Design review of the part built by this model. Coordinates are the model's own, in mm. Give positions to 0.01 mm unless a question says otherwise; leave off trailing zeros. Order: outer loops, then holes, each group sorted by start corner. A loop starts at its lowest first (then second) coordinate and runs counter-clockwise, first axis right, second up.
```python
from build123d import *

# Parameters (mm, degrees)
SKICA1_R                     = 76.5
P_IDAT_VYSUNUT_M1_DEPTH      = 20
P_IDAT_VYSUNUT_M1_DEPTH_BACK = 6.6
ODEBRAT_VYSUNUT_M1_DEPTH     = 5
ZAOBLIT1_R                   = 2
ZAOBLIT2_R                   = 5


with BuildPart() as part:
    # Skica1 → Přidat vysunutím1 (new body, two sides)
    with BuildSketch(Plane.XY) as p_idat_vysunut_m1_sk:
        Circle(SKICA1_R)
    extrude(amount=P_IDAT_VYSUNUT_M1_DEPTH)
    extrude(p_idat_vysunut_m1_sk.sketch, amount=-P_IDAT_VYSUNUT_M1_DEPTH_BACK)

    # Skica2 → Odebrat vysunutím1 (cut)
    with BuildSketch(Plane(origin=(0, 0, -6.6), x_dir=(-1, 0, 0), z_dir=(0, 0, -1))):
        Polygon((25, -10), (48.8, -10), (48.8, 10), (25, 10), (25, 25), (10, 25), (10, 48.8), (-10, 48.8), (-10, 25), (-25, 25), (-25, 10), (-48.8, 10), (-48.8, -10), (-25, -10), (-25, -25), (-10, -25), (-10, -48.8), (10, -48.8), (10, -25), (25, -25), align=None)
    extrude(amount=-ODEBRAT_VYSUNUT_M1_DEPTH, mode=Mode.SUBTRACT)

    # Zaoblit1
    zaoblit1_edges = [part.edges().sort_by_distance(p)[0] for p in [
        (-25, -17.5, -6.6),
        (-36.9, -10, -6.6),
        (-48.8, 0, -6.6),
        (-36.9, 10, -6.6),
        (-25, 17.5, -6.6),
        (-17.5, 25, -6.6),
        (-10, 36.9, -6.6),
        (0, 48.8, -6.6),
        (10, 36.9, -6.6),
        (17.5, 25, -6.6),
        (25, 17.5, -6.6),
        (36.9, 10, -6.6),
        (48.8, 0, -6.6),
        (36.9, -10, -6.6),
        (25, -17.5, -6.6),
        (17.5, -25, -6.6),
        (10, -36.9, -6.6),
        (0, -48.8, -6.6),
        (-10, -36.9, -6.6),
        (-17.5, -25, -6.6),
    ]]
    fillet(zaoblit1_edges, radius=ZAOBLIT1_R)

    # Zaoblit2
    zaoblit2_edges = [part.edges().sort_by_distance(p)[0] for p in [
        (-76.5, 0, 20),
        (-76.5, 0, -6.6),
    ]]
    fillet(zaoblit2_edges, radius=ZAOBLIT2_R)


solid = part.part
```
1. For line 1 along Y through (x, z) = (27, -4.25); line 2 along Z through (x, y) = (-2.5, -30); line 3 along Y through (x, z) = (34.5, -4.25), list the stretches that pass through material, from the lowest coordinate up.
Recorded:
line 1: y = -70.76 to -10, 10 to 70.76
line 2: z = -1.6 to 20
line 3: y = -67.43 to -10, 10 to 67.43
2. For pin 1 (10 mm diameter, centred on x = 34, z = 10.5, fed in from +Y); pin 2 (2.5 mm diameter, centred on x = -3.5, z = -3, fed in from -Y); pin 3 (1.5 mm diameter, centred on x = -43, z = -3, fed in from -Y); pin 4 (6 mm diameter, centred on y = 2, z = 13.5, fed in from -X), all flat-tipped, find the tip position at first contact; note any pin that passes through.
Recorded:
pin 1: stops at y = 70.79
pin 2: stops at y = -76.44
pin 3: stops at y = -63.59
pin 4: stops at x = -76.5
3. Take a section at A-A (x = 0). State the section outline as (y, z) points, then the cut area to 3 significant figures.
Recorded:
outline: (-76.5, -1.6) arc R5 ccw to (-71.5, -6.6) - (-50.8, -6.6) arc R2 ccw to (-48.8, -4.6) - (-48.8, -1.6) - (48.8, -1.6) - (48.8, -4.6) arc R2 ccw to (50.8, -6.6) - (71.5, -6.6) arc R5 ccw to (76.5, -1.6) - (76.5, 15) arc R5 ccw to (71.5, 20) - (-71.5, 20) arc R5 ccw to (-76.5, 15) - close
area: 3,560 mm2
4. Draft analysis for pull direction Y (two halves, no side actions). For faces 1 (the face through (1, 1, -1.6)), 2 (the face through (-60.708, -46.549, 6.816)), 3 (the face through (15, -31, -6.6)), state which applies: pulls with the +Y half, pulls with the -Y half, needs draft (parallel to the pull), parting line crosses it, or undercut.
Recorded:
face 1: undercut
face 2: parting line crosses it
face 3: needs draft
5. Take a section at C-C (z = 4). State the section outline as (x, y) points.
Recorded:
outline: circle Ø153 at (0, 0)
